```python
from build123d import *

# Parameters (mm, degrees)
SKETCH1_W           = 450
SKETCH1_H           = 210
BOSS_EXTRUDE1_DEPTH = 5
SKETCH3_W           = 65.821391225
SKETCH3_H           = 25
SKETCH3_W_2         = 143.228691138
SKETCH3_H_2         = 30
SKETCH3_W_3         = 192.205874683
SKETCH3_W_4         = 194.707934706
SKETCH3_W_5         = 70.821391225
SKETCH3_W_6         = 148.228691138
SKETCH3_W_7         = 194.705874683
SKETCH3_W_8         = 199.707934706
CUT_EXTRUDE1_DEPTH  = 6


with BuildPart() as part:
    # Sketch1 → Boss-Extrude1 (new body)
    with BuildSketch(Plane.XY):
        Rectangle(SKETCH1_W, SKETCH1_H)
    extrude(amount=BOSS_EXTRUDE1_DEPTH)

    # Sketch3 → Cut-Extrude1 (cut, through all)
    with BuildSketch(Plane(origin=(0, 0, 0), x_dir=(-1, 0, 0), z_dir=(0, 0, -1))):
        with Locations((-252.910695613, 92.5)):
            Rectangle(SKETCH3_W, SKETCH3_H)
        with Locations((-291.614345569, 35)):
            Rectangle(SKETCH3_W_2, SKETCH3_H_2)
        with Locations((-316.102937342, -25)):
            Rectangle(SKETCH3_W_3, SKETCH3_H_2)
        with Locations((-317.353967353, -82.5)):
            Rectangle(SKETCH3_W_4, SKETCH3_H)
        with Locations((255.410695613, 92.5)):
            Rectangle(SKETCH3_W_5, SKETCH3_H)
        with Locations((294.114345569, 35)):
            Rectangle(SKETCH3_W_6, SKETCH3_H_2)
        with Locations((317.352937342, -25)):
            Rectangle(SKETCH3_W_7, SKETCH3_H_2)
        with Locations((319.853967353, -82.5)):
            Rectangle(SKETCH3_W_8, SKETCH3_H)
    extrude(amount=-CUT_EXTRUDE1_DEPTH, mode=Mode.SUBTRACT)


solid = part.part
```
CAD build for the part. Positions are in the model's coordinates, mm. Round coordinates to 2 decimals unless told otherwise and drop trailing zeros. Order: outer loops, then holes, each group sorted by start corner. A loop starts at its lowest first (then second) coordinate and runs counter-clockwise, first axis right, second up.
Q1. Slice it at A-A (y = -21.5). Write the cut outline in (x, z).
Q2. Wall check: L1, parallel to X at y = 80.5, z = 4.4. Give the ranges that are in metal, low to high.
Q3. Drop flat-ended pins along their axis: pin 1 (2.5 mm diameter, centred on y = 96, z = 2.5, fed in from +X); pin 2 (1 mm diameter, centred on x = 24, y = 60, fed in from -Z); pin 3 (2.5 mm diameter, centred on x = -222.5, z = 2, fed in from +Y); pin 4 (1.5 mm diameter, centred on y = -20, z = 1.5, fed in from -X). Give the stop position or say it passes through.
Results below:
1. outline: (-220, 0) - (220, 0) - (220, 5) - (-220, 5) - close
2. L1: x = -220 to 220
3. pin 1: stops at x = 220
3. pin 2: stops at z = 0
3. pin 3: stops at y = 80
3. pin 4: stops at x = -220
